```python
from build123d import *

# Parameters (mm, degrees)
F1_DEPTH = 13.2
F2_T     = -1.6
F4_D     = 7


with BuildPart() as f1:
    # F0 (on Front) → F1 (new body)
    with BuildSketch(Plane.XZ):
        with BuildLine():
            Line((-8.349, 15.907), (-8.349, 0))
            Line((-8.349, 0), (8.349, 0))
            Line((8.349, 0), (8.349, 15.907))
            ThreePointArc((8.349, 15.907), (7.5895278836, 17.7405278836), (5.756, 18.5))
            Line((5.756, 18.5), (-5.756, 18.5))
            ThreePointArc((-5.756, 18.5), (-7.5895278836, 17.7405278836), (-8.349, 15.907))
        make_face()
    extrude(amount=F1_DEPTH)

    # F2
    f2_openings = [f1.faces().sort_by_distance(p)[0] for p in [
        (0, -6.6, 0),
    ]]
    offset(amount=F2_T, openings=f2_openings)

    # F4 (through all)
    with Locations(Plane.XY.offset(18.5)):
        with Locations((0, -6.6)):
            Hole(F4_D / 2)


solid = f1.part
```
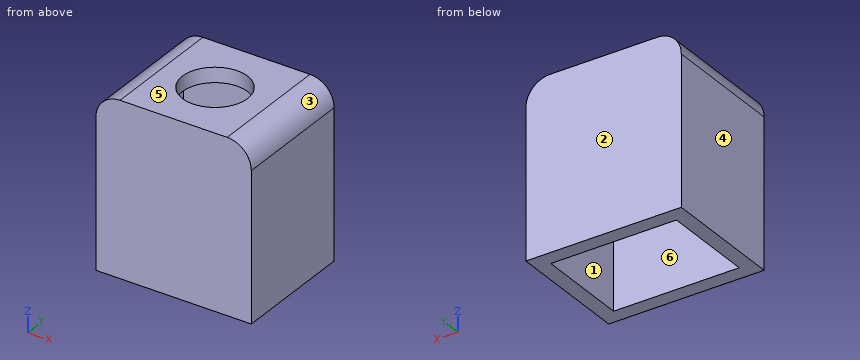
Design review of the part built by this model. Coordinates are the model's own, in mm. Face numbers are marked on the shaded views. A direction names the side the tool comes from. Coordinates: 2 decimals unless noted, no trailing zeros. Order: outer loops, then holes, each group sorted by start corner. A loop starts at its lowest first (then second) coordinate and runs counter-clockwise, first axis right, second up. Notation, with made-up numbers: (18, 76.5) -> (74, 76.5) arc R13 ccw to (74, 99.5) -> close; hole circle Ø9 at (71, 22). An arc over 180 degrees is marked (long way). One line per item, written item: value. Start each with the question number.
Q1. For probe 1 along Y at (x, z) = (-1.5, 4.75); probe 2 along X at (y, z) = (-4, 14.25); probe 3 along Y at (x, z) = (0, 17.7), list the stretches that pass through material, from the lowest coordinate up.
Q2. Take a section at C-C, the plane z = 15.25. State the section outline as (x, y) points, then the cut area to 3 significant figures.
Q3. Mouldability with a two-part tool opening along X and no side actions: class the marked faces 1, 2, 3 and 4 as pulls with the +X half, pulls with the -X half, needs draft (parallel to the pull), parting line crosses it, or undercut.
Q4. Insertion check: pin 1 Ø6 at (x, z) = (-2, 14.5) entering from +Y; pin 2 Ø5 at (x, y) = (-0.5, -5.5) entering from -Z. Each pin has a flat end and moves straight along its axis. Give the tip position at first contact, or say it passes through.
Q5. Take a section at D-D, the plane x = -4. State the section outline as (y, z) points, then the cut area to 3 significant figures.
Q6. Take a section at A-A, the plane y = -6.6. State the section outline as (x, z) points, then the cut area to 3 significant figures.
Q7. Take a section at B-B, the plane x = 0. State the section outline as (y, z) points, then the cut area to 3 significant figures.
Q8. Tool access review of the marked faces 5 and 6: name each direction out of +Z, -Z, +X, -X, +Y, -Y from which nothing blocks a thin tool from reaching the whole face with its end or side.
Values follow:
1. probe 1: y = -13.2 to -11.6, -1.6 to 0
1. probe 2: x = -8.35 to -6.75, 6.75 to 8.35
1. probe 3: y = -13.2 to -10.1, -3.1 to 0
2. outline: (-8.35, -13.2) -> (8.35, -13.2) -> (8.35, 0) -> (-8.35, 0) -> close; hole (-6.75, -11.6) -> (6.75, -11.6) -> (6.75, -1.6) -> (-6.75, -1.6) -> close
2. area: 85.4 mm2
3. face 1: undercut
3. face 2: needs draft
3. face 3: pulls with the +X half
3. face 4: pulls with the -X half
4. pin 1: stops at y = 0
4. pin 2: stops at z = 16.9
5. outline: (-13.2, 0) -> (-11.6, 0) -> (-11.6, 16.9) -> (-1.6, 16.9) -> (-1.6, 0) -> (0, 0) -> (0, 18.5) -> (-13.2, 18.5) -> close
5. area: 75.2 mm2
6. outline: (-8.35, 0) -> (-6.75, 0) -> (-6.75, 15.91) arc R0.99 cw to (-5.76, 16.9) -> (-3.5, 16.9) -> (-3.5, 18.5) -> (-5.76, 18.5) arc R2.59 ccw to (-8.35, 15.91) -> close; (3.5, 16.9) -> (5.76, 16.9) arc R0.99 cw to (6.75, 15.91) -> (6.75, 0) -> (8.35, 0) -> (8.35, 15.91) arc R2.59 ccw to (5.76, 18.5) -> (3.5, 18.5) -> close
6. area: 67.1 mm2
7. outline: (-13.2, 0) -> (-11.6, 0) -> (-11.6, 16.9) -> (-10.1, 16.9) -> (-10.1, 18.5) -> (-13.2, 18.5) -> close; (-3.1, 16.9) -> (-1.6, 16.9) -> (-1.6, 0) -> (0, 0) -> (0, 18.5) -> (-3.1, 18.5) -> close
7. area: 64.0 mm2
8. face 5: +Z, +X, -X, +Y, -Y
8. face 6: -Z
